```python
from build123d import *

# Parameters (mm, degrees)
BOSS_EXTRUDE1_DEPTH = 26
CUT_EXTRUDE1_REACH  = 64.658
SKETCH2_R           = 1.6
CUT_EXTRUDE5_REACH  = 63.563
SKETCH6_R           = 1.6
FILLET1_R           = 1
CUT_EXTRUDE6_REACH  = 64.658
FILLET2_R           = 10


with BuildPart() as part:
    # Sketch1 → Boss-Extrude1 (new, symmetric)
    with BuildSketch(Plane(origin=(0, 0, 0), x_dir=(0, 0, -1), z_dir=(1, 0, 0))):
        Polygon((0, -45), (0, 45), (35, 45), (35, 35), (33, 35), (33, 43), (2, 43), (2, -43), (33, -43), (33, -35), (35, -35), (35, -45), align=None)
    extrude(amount=BOSS_EXTRUDE1_DEPTH, both=True)

    # Sketch2 → Cut-Extrude1 (cut, up to next)
    with BuildSketch(Plane.XY, mode=Mode.PRIVATE) as cut_extrude1_sk1:
        with Locations((-21, -39)):
            Circle(SKETCH2_R)
    cut_extrude1_tool1 = extrude(cut_extrude1_sk1.sketch, amount=-CUT_EXTRUDE1_REACH, mode=Mode.PRIVATE) & part.part
    # Sketch2 → Cut-Extrude1 (cut, up to next)
    with BuildSketch(Plane.XY, mode=Mode.PRIVATE) as cut_extrude1_sk2:
        with Locations((-21, 39)):
            Circle(SKETCH2_R)
    cut_extrude1_tool2 = extrude(cut_extrude1_sk2.sketch, amount=-CUT_EXTRUDE1_REACH, mode=Mode.PRIVATE) & part.part
    # Sketch2 → Cut-Extrude1 (cut, up to next)
    with BuildSketch(Plane.XY, mode=Mode.PRIVATE) as cut_extrude1_sk3:
        with Locations((21, 39)):
            Circle(SKETCH2_R)
    cut_extrude1_tool3 = extrude(cut_extrude1_sk3.sketch, amount=-CUT_EXTRUDE1_REACH, mode=Mode.PRIVATE) & part.part
    # Sketch2 → Cut-Extrude1 (cut, up to next)
    with BuildSketch(Plane.XY, mode=Mode.PRIVATE) as cut_extrude1_sk4:
        with Locations((21, -39)):
            Circle(SKETCH2_R)
    cut_extrude1_tool4 = extrude(cut_extrude1_sk4.sketch, amount=-CUT_EXTRUDE1_REACH, mode=Mode.PRIVATE) & part.part
    add(cut_extrude1_tool1.solids().sort_by_distance((-21, -39, 0))[0], mode=Mode.SUBTRACT)
    add(cut_extrude1_tool2.solids().sort_by_distance((-21, 39, 0))[0], mode=Mode.SUBTRACT)
    add(cut_extrude1_tool3.solids().sort_by_distance((21, 39, 0))[0], mode=Mode.SUBTRACT)
    add(cut_extrude1_tool4.solids().sort_by_distance((21, -39, 0))[0], mode=Mode.SUBTRACT)

    # Sketch6 → Cut-Extrude5 (cut, up to next)
    with BuildSketch(Plane.XY.offset(-33), mode=Mode.PRIVATE) as cut_extrude5_sk1:
        with Locations((16, -39)):
            Circle(SKETCH6_R)
    cut_extrude5_tool1 = extrude(cut_extrude5_sk1.sketch, amount=-CUT_EXTRUDE5_REACH, mode=Mode.PRIVATE) & part.part
    # Sketch6 → Cut-Extrude5 (cut, up to next)
    with BuildSketch(Plane.XY.offset(-33), mode=Mode.PRIVATE) as cut_extrude5_sk2:
        with Locations((-16, -39)):
            Circle(SKETCH6_R)
    cut_extrude5_tool2 = extrude(cut_extrude5_sk2.sketch, amount=-CUT_EXTRUDE5_REACH, mode=Mode.PRIVATE) & part.part
    # Sketch6 → Cut-Extrude5 (cut, up to next)
    with BuildSketch(Plane.XY.offset(-33), mode=Mode.PRIVATE) as cut_extrude5_sk3:
        with Locations((-16, 39)):
            Circle(SKETCH6_R)
    cut_extrude5_tool3 = extrude(cut_extrude5_sk3.sketch, amount=-CUT_EXTRUDE5_REACH, mode=Mode.PRIVATE) & part.part
    # Sketch6 → Cut-Extrude5 (cut, up to next)
    with BuildSketch(Plane.XY.offset(-33), mode=Mode.PRIVATE) as cut_extrude5_sk4:
        with Locations((16, 39)):
            Circle(SKETCH6_R)
    cut_extrude5_tool4 = extrude(cut_extrude5_sk4.sketch, amount=-CUT_EXTRUDE5_REACH, mode=Mode.PRIVATE) & part.part
    add(cut_extrude5_tool1.solids().sort_by_distance((16, -39, -33))[0], mode=Mode.SUBTRACT)
    add(cut_extrude5_tool2.solids().sort_by_distance((-16, -39, -33))[0], mode=Mode.SUBTRACT)
    add(cut_extrude5_tool3.solids().sort_by_distance((-16, 39, -33))[0], mode=Mode.SUBTRACT)
    add(cut_extrude5_tool4.solids().sort_by_distance((16, 39, -33))[0], mode=Mode.SUBTRACT)

    # Fillet1
    fillet1_edges = [part.edges().sort_by_distance(p)[0] for p in [
        (0, 43, -33),
        (0, 43, -2),
        (0, -43, -2),
        (0, -43, -33),
    ]]
    fillet(fillet1_edges, radius=FILLET1_R)

    # Sketch7 → Cut-Extrude6 (cut, up to next)
    with BuildSketch(Plane.XY, mode=Mode.PRIVATE) as cut_extrude6_sk1:
        Polygon((-26, 30), (-18, 25), (-18, -25), (-26, -30), align=None)
    cut_extrude6_tool1 = extrude(cut_extrude6_sk1.sketch, amount=-CUT_EXTRUDE6_REACH, mode=Mode.PRIVATE) & part.part
    # Sketch7 → Cut-Extrude6 (cut, up to next)
    with BuildSketch(Plane.XY, mode=Mode.PRIVATE) as cut_extrude6_sk2:
        Polygon((26, -30), (18, -25), (18, 25), (26, 30), align=None)
    cut_extrude6_tool2 = extrude(cut_extrude6_sk2.sketch, amount=-CUT_EXTRUDE6_REACH, mode=Mode.PRIVATE) & part.part
    add(cut_extrude6_tool1.solids().sort_by_distance((-22.121212, 0, 0))[0], mode=Mode.SUBTRACT)
    add(cut_extrude6_tool2.solids().sort_by_distance((22.121212, 0, 0))[0], mode=Mode.SUBTRACT)

    # Fillet2
    fillet2_edges = [part.edges().sort_by_distance(p)[0] for p in [
        (18, -25, -1),
        (18, 25, -1),
        (-18, 25, -1),
        (-18, -25, -1),
    ]]
    fillet(fillet2_edges, radius=FILLET2_R)


solid = part.part
```
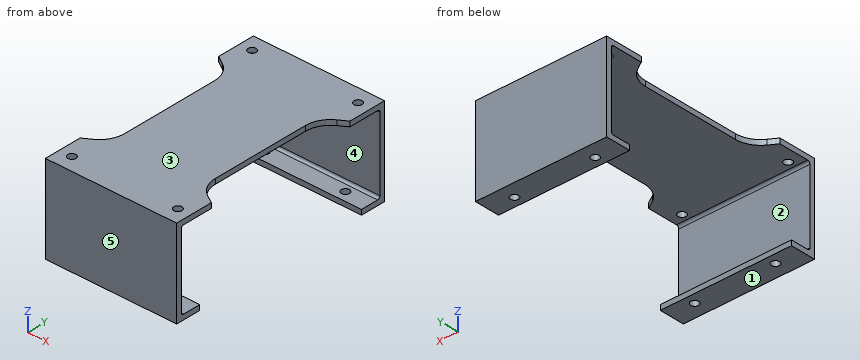
Could you check a few things on this model? Use its own coordinates, in mm. Face numbers are marked on the shaded views. A direction names the side the tool comes from. Give positions to 0.01 mm unless a question says otherwise; leave off trailing zeros. Write each loop counter-clockwise with the first axis right and the second up, starting at its lowest first coordinate (ties: lowest second). Pieces come first, ordered by that corner, then holes. Notation, with made-up numbers: (-32, 39.5) - (19, 39.5) arc R16 cw to (19, 45.5) - close; hole circle Ø1 at (54, -9.5). An arc over 180 degrees is marked (long way). One line per item, written item: value. Start each with the question number.
Item 1: I'm going to push flat-ended pins straight in: pin 1 (5 mm diameter, centred on x = 13.5, y = 26.5, fed in from -Z); pin 2 (1.6 mm diameter, centred on y = -8.5, z = -1, fed in from -X). Where does each tip first touch, or does it pass through?
Item 2: Imagine slicing it at C-C, the plane z = -9. List the corners of the cut face in (x, y) for me, and give its area (3 significant figures).
Item 3: Imagine slicing it at B-B, the plane x = -16. List the corners of the cut face in (y, z) for me, and give its area (3 significant figures).
Item 4: Please list where these lines run through material, in increasing order: line 1 (Y direction, x = 16, z = -34); line 2 (Y direction, x = -5, z = -29); line 3 (Y direction, x = -21, z = -0.95). Write a range as from..to.
Item 5: If we mould it in two halves opening along Z, with no side actions, what happens to the marked faces 3, 4 and 5? For each: +Z half, -Z half, draft (parallel to the pull), parting line (faces both ways), or undercut.
Item 6: Which directions (+Z, -Z, +X, -X, +Y, -Y) give clear straight access to the entire face, cutting with the end or side of a thin tool? Please do the marked faces 1 and 2.
Item 7: Imagine slicing it at D-D, the plane x = -10.5. List the corners of the cut face in (y, z) for me, and give its area (3 significant figures).
Item 8: Imagine slicing it at A-A, the plane y = 39. List the corners of the cut face in (x, z) for me.
Geometry says:
1. pin 1: z = -2
1. pin 2: x = -18
2. outline: (-26, -45) - (26, -45) - (26, -43) - (-26, -43) - close; (-26, 43) - (26, 43) - (26, 45) - (-26, 45) - close
2. area: 208 mm^2
3. outline: (-45, -35) - (-40.6, -35) - (-40.6, -33) - (-42, -33) arc R1 cw to (-43, -32) - (-43, -3) arc R1 cw to (-42, -2) - (42, -2) arc R1 cw to (43, -3) - (43, -32) arc R1 cw to (42, -33) - (40.6, -33) - (40.6, -35) - (45, -35) - (45, 0) - (-45, 0) - close; (-37.4, -35) - (-35, -35) - (-35, -33) - (-37.4, -33) - close; (35, -35) - (37.4, -35) - (37.4, -33) - (35, -33) - close
3. area: 332 mm^2
4. line 1: -45..-40.6, -37.4..-35, 35..37.4, 40.6..45
4. line 2: -45..-43, 43..45
4. line 3: -45..-40.6, -37.4..-26.6, 26.6..37.4, 40.6..45
5. face 3: +Z half
5. face 4: undercut
5. face 5: draft
6. face 1: -Z, +X, -X, +Y, -Y
6. face 2: +X, -X
7. outline: (-45, -35) - (-35, -35) - (-35, -33) - (-42, -33) arc R1 cw to (-43, -32) - (-43, -3) arc R1 cw to (-42, -2) - (42, -2) arc R1 cw to (43, -3) - (43, -32) arc R1 cw to (42, -33) - (35, -33) - (35, -35) - (45, -35) - (45, 0) - (-45, 0) - close
7. area: 345 mm^2
8. outline: (-26, -35) - (-17.6, -35) - (-17.6, -33) - (-26, -33) - close; (-26, -2) - (-22.6, -2) - (-22.6, 0) - (-26, 0) - close; (-19.4, -2) - (19.4, -2) - (19.4, 0) - (-19.4, 0) - close; (-14.4, -35) - (14.4, -35) - (14.4, -33) - (-14.4, -33) - close; (17.6, -35) - (26, -35) - (26, -33) - (17.6, -33) - close; (22.6, -2) - (26, -2) - (26, 0) - (22.6, 0) - close
